Source: CAD feature listing. Evaluate the final solid. Frame: model axes, mm. A direction names the side the tool comes from. Round coordinates to 2 decimals unless told otherwise and drop trailing zeros. Order: outer loops, then holes, each group sorted by start corner. A loop starts at its lowest first (then second) coordinate and runs counter-clockwise, first axis right, second up. Notation, with made-up numbers: M -5,89.5 L 44,89.5 A18 cw 44,101.5 Z; hole C 35.25,-15.5 d5. An arc over 180 degrees is marked long. Answer in a Markdown table with one row per item. Add a question column.
```python
from build123d import *

# Parameters (mm, degrees)
F0_R     = 4.95
F0_R_2   = 2.45
F1_DEPTH = 4
F2_W     = 0.722248
F2_H     = 1.3
F2_W_2   = 0.566372


with BuildPart() as f1:
    # F0 (on Front) → F1 (new body)
    with BuildSketch(Plane.XZ):
        Circle(F0_R)
        Circle(F0_R_2, mode=Mode.SUBTRACT)
    extrude(amount=F1_DEPTH)

    # F2 (on Right) → F3 (revolve, cut)
    with BuildSketch(Plane.YZ):
        with Locations((-4.061124, 3.75)):
            Rectangle(F2_W, F2_H)
        with Locations((-0.016814, 3.75)):
            Rectangle(F2_W_2, F2_H)
    revolve(axis=Axis((0, -1, 0), (0, -1, 0)), mode=Mode.SUBTRACT)


solid = f1.part
```
(1) Cut plane A-A (x = 0). Return loops of the section in (y, z).
(2) Line query: line 1 (Z direction, x = 0, y = -3.9); line 2 (Z direction, x = -0.25, y = -0.9); line 3 (Z direction, x = -2, y = -0.5). Output: solid intervals per line, ascending. Write a range as from..to.
(3) Pin query (flat end, axial travel): pin 1 (4 mm diameter, centred on x = 4, z = 1, fed in from +Y); pin 2 (4.5 mm diameter, centred on x = 0, z = 0, fed in from -Y). Return the tip coordinate at first contact, or that it passes through.
(4) Draft query along X for faces 3 (the face through (4.72, -1.97, 1.49)), 4 (the face through (-0.5, -2, -2.4)). Return one class per face: +X half, -X half, draft (parallel to the pull), parting line (faces both ways), or undercut.
(5) Cut plane B-B (z = 0). Return loops of the section in (x, y).
(6) Access query for faces 1 (the face through (3, -0.3, -2)), 2 (the face through (3, -3.7, -2)). Directions: +Z, -Z, +X, -X, +Y, -Y. A direction counts if a zero-diameter tool reaches every point of the face in a straight line with its end or side. Return the directions, or none.
(7) Cut plane D-D (x = 4). Return loops of the section in (y, z).
(8) Cut plane C-C (y = -2.8). Return loops of the section in (x, z), and give its area (3 significant figures).
Answer list:
| question | item | result |
|---|---|---|
| 1 | outline | M -4,-4.95 L 0,-4.95 L 0,-4.4 L -0.3,-4.4 L -0.3,-3.1 L 0,-3.1 L 0,-2.45 L -4,-2.45 L -4,-3.1 L -3.7,-3.1 L -3.7,-4.4 L -4,-4.4 Z; M -4,2.45 L 0,2.45 L 0,3.1 L -0.3,3.1 L -0.3,4.4 L 0,4.4 L 0,4.95 L -4,4.95 L -4,4.4 L -3.7,4.4 L -3.7,3.1 L -4,3.1 Z |
| 2 | line 1 | -4.95..-4.4, -3.1..-2.45, 2.45..3.1, 4.4..4.95 |
| 2 | line 2 | -4.94..-2.44, 2.44..4.94 |
| 2 | line 3 | -4.53..-1.42, 1.42..4.53 |
| 3 | pin 1 | y = 0 |
| 3 | pin 2 | through |
| 4 | face 3 | parting line |
| 4 | face 4 | undercut |
| 5 | outline | M -4.95,-4 L -4.4,-4 L -4.4,-3.7 L -3.1,-3.7 L -3.1,-4 L -2.45,-4 L -2.45,0 L -3.1,0 L -3.1,-0.3 L -4.4,-0.3 L -4.4,0 L -4.95,0 Z; M 2.45,-4 L 3.1,-4 L 3.1,-3.7 L 4.4,-3.7 L 4.4,-4 L 4.95,-4 L 4.95,0 L 4.4,0 L 4.4,-0.3 L 3.1,-0.3 L 3.1,0 L 2.45,0 Z |
| 6 | face 1 | +Y |
| 6 | face 2 | -Y |
| 7 | outline | M -4,-2.92 L 0,-2.92 L 0,-1.83 L -0.3,-1.83 L -0.3,1.83 L 0,1.83 L 0,2.92 L -4,2.92 L -4,1.83 L -3.7,1.83 L -3.7,-1.83 L -4,-1.83 Z |
| 8 | outline | C 0,0 d9.9; hole C 0,0 d4.9 |
| 8 | area | 58.1 mm² |
